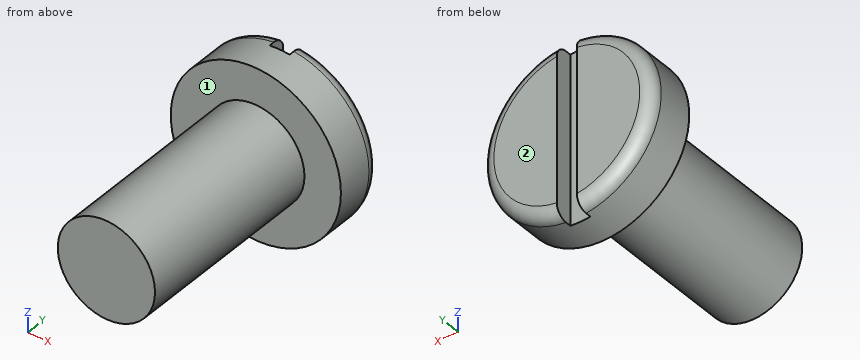
```python
from build123d import *

# Parameters (mm, degrees)
SKETCH1_R               = 3.5
SKETCH1_R_2             = 2
BOSS_EXTRUDE1_DEPTH     = 2
SKETCH1_2_R             = 2
BOSS_EXTRUDE2_DEPTH     = 10
SKETCH2_W               = 0.824993444
SKETCH2_H               = 1.453522708
CUT_EXTRUDE1_DEPTH      = 4.5
CUT_EXTRUDE1_DEPTH_BACK = 4.5
FILLET2_R               = 0.5


with BuildPart() as part:
    # Sketch1 → Boss-Extrude1 (new body)
    with BuildSketch(Plane(origin=(0, 0, 0), x_dir=(1, 0, 0), z_dir=(0, 1, 0))):
        Circle(SKETCH1_R)
        Circle(SKETCH1_R_2, mode=Mode.SUBTRACT)
    extrude(amount=-BOSS_EXTRUDE1_DEPTH)

    # Sketch1<2> → Boss-Extrude2 (add)
    with BuildSketch(Plane(origin=(0, 0, 0), x_dir=(1, 0, 0), z_dir=(0, 1, 0))):
        Circle(SKETCH1_2_R)
    extrude(amount=-BOSS_EXTRUDE2_DEPTH)

    # Sketch2 → Cut-Extrude1 (cut, two sides)
    with BuildSketch(Plane.XY) as cut_extrude1_sk:
        Rectangle(SKETCH2_W, SKETCH2_H)
    extrude(amount=CUT_EXTRUDE1_DEPTH, mode=Mode.SUBTRACT)
    extrude(cut_extrude1_sk.sketch, amount=-CUT_EXTRUDE1_DEPTH_BACK, mode=Mode.SUBTRACT)

    # Fillet2
    fillet2_edges = [part.edges().sort_by_distance(p)[0] for p in [
        (2.616652301, 0, -2.324463537),
        (-3.5, 0, 0),
    ]]
    fillet(fillet2_edges, radius=FILLET2_R)


solid = part.part
```
Geometry: final body of the model. Coordinates: model frame, mm. Face numbers are marked on the shaded views. A direction names the side the tool comes from. Round coordinates to 2 decimals unless told otherwise and drop trailing zeros. Write each loop counter-clockwise with the first axis right and the second up, starting at its lowest first coordinate (ties: lowest second). Pieces come first, ordered by that corner, then holes.
Item 1: Section query B-B (x = 0). Return loops of the section in (y, z).
Item 2: Section query A-A (z = 0). Return loops of the section in (x, y), plus the area to 3 significant figures.
Item 3: Set-up query: the marked faces 1 and 2. Return all of +Z, -Z, +X, -X, +Y, -Y with unobstructed straight access to the full face (end or side cutting, diameter ignored); none if empty.
Item 4: Pin query (flat end, axial travel): P1, Ø0.8, axis at y = -0.5, z = 1.5, coming from the +X side; P2, Ø4, axis at x = 1, y = -4.5, coming from the -Z side; P3, Ø4, axis at y = -3.5, z = -1.5, coming from the -X side. Return the tip coordinate at first contact, or that it passes through.
Item 5: Material intervals for L1, parallel to Y at x = -2.5, z = -0.25; L2, parallel to X at y = -8.75, z = 0; L3, parallel to X at y = -2.5, z = 0.75, sorted ascending.
Item 6: Section query D-D (y = -5.5). Return loops of the section in (x, z).
Item 7: Section query C-C (y = -1.25). Return loops of the section in (x, z), plus the area to 3 significant figures.
Completed:
1. outline: (-10, -2) - (-2, -2) - (-2, -3.5) - (-0.73, -3.5) - (-0.73, 3.5) - (-2, 3.5) - (-2, 2) - (-10, 2) - close
2. outline: (-3.5, -2) - (-2, -2) - (-2, -10) - (2, -10) - (2, -2) - (3.5, -2) - (3.5, -0.5) arc R0.5 ccw to (3, 0) - (0.41, 0) - (0.41, -0.73) - (-0.41, -0.73) - (-0.41, 0) - (-3, 0) arc R0.5 ccw to (-3.5, -0.5) - close
2. area: 45.3 mm2
3. face 1: -Y
3. face 2: +Z, -Z, +X, -X, +Y
4. P1: stops at x = 3.32
4. P2: stops at z = -2
4. P3: stops at x = -3.5
5. L1: y = -2 to 0
5. L2: x = -2 to 2
5. L3: x = -1.85 to 1.85
6. outline: circle Ø4 at (0, 0)
7. outline: circle Ø7 at (0, 0)
7. area: 38.5 mm2
